Part print with two shaded views. Sizes in mm from the minimum x, y, z corner. A direction names the side the tool comes from. Coordinates: 2 decimals unless noted, no trailing zeros. Loops run counter-clockwise (first coordinate to the right, second up) from the corner with the lowest first, then second, coordinate; pieces in that order, holes last.
Item 1: 3-axis set-ups, long thin cutter, end or side, ignore diameter. For the marked faces 1, 2 and 3: which of +Z, -Z, +X, -X, +Y, -Y reach the whole face in a straight line?
Item 2: Flat gauge pins, fed straight in: pin 1 (10 mm diameter, centred on y = 8.5, z = 47.5, fed in from -X); pin 2 (10 mm diameter, centred on x = 39.5, z = 40.5, fed in from +Y); pin 3 (4 mm diameter, centred on y = 2, z = 29, fed in from -X). Where does each tip first touch, or does it go through?
Item 3: Cut at B-B (y = 17.75). List the corners of the cut face in (x, z).
Item 4: Drill centre lines: line 1 along Z through (x, y) = (29, 17); line 2 along Y through (x, z) = (24.5, 40.5). Where is each one in solid material? Low to high.
Item 5: Cut at A-A (z = 29). List the corners of the cut face in (x, y), and give its area (3 significant figures).
Item 6: Cut at D-D (y = 14.75). List the corners of the cut face in (x, z), and give its area (3 significant figures).
Item 7: Cut at C-C (x = 29). List the corners of the cut face in (y, z), and give its area (3 significant figures).
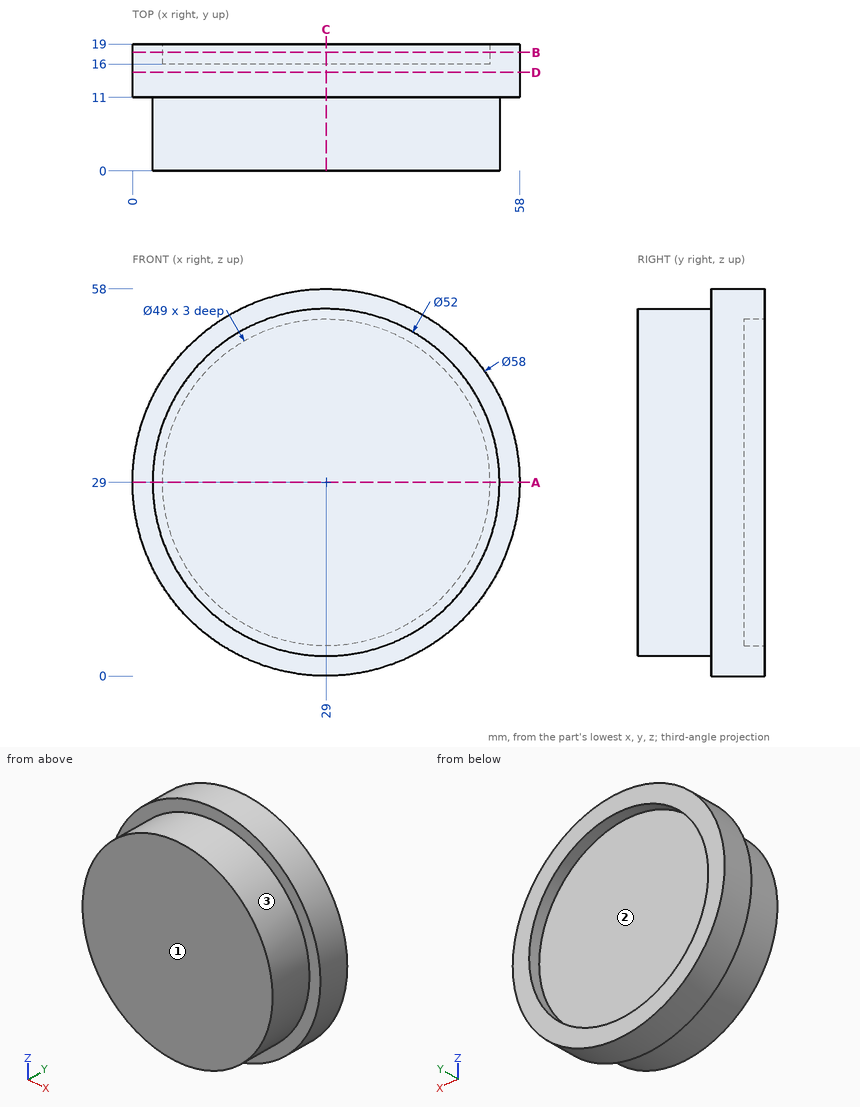
Filled sheet:
1. face 1: +Z, -Z, +X, -X, -Y
1. face 2: +Y
1. face 3: -Y
2. pin 1: stops at x = 3.7
2. pin 2: stops at y = 16
2. pin 3: stops at x = 3
3. outline: circle Ø58 at (29, 29); hole circle Ø49 at (29, 29)
4. line 1: z = 0 to 4.5, 53.5 to 58
4. line 2: y = 0 to 16
5. outline: (0, 11) - (3, 11) - (3, 0) - (55, 0) - (55, 11) - (58, 11) - (58, 19) - (53.5, 19) - (53.5, 16) - (4.5, 16) - (4.5, 19) - (0, 19) - close
5. area: 889 mm2
6. outline: circle Ø58 at (29, 29)
6. area: 2,640 mm2
7. outline: (0, 3) - (11, 3) - (11, 0) - (19, 0) - (19, 4.5) - (16, 4.5) - (16, 53.5) - (19, 53.5) - (19, 58) - (11, 58) - (11, 55) - (0, 55) - close
7. area: 889 mm2
